Verification items for the finished model (mm, model axes). Round coordinates to 2 decimals unless told otherwise and drop trailing zeros. Loops run counter-clockwise (first coordinate to the right, second up) from the corner with the lowest first, then second, coordinate; pieces in that order, holes last. Notation, with made-up numbers: (76.25, -39) - (111.25, -39) arc R25 ccw to (111.25, -17) - close; hole circle Ø8 at (0.5, 43.25). An arc over 180 degrees is marked (long way). Use CSV: the item, a comma, the result in double quotes.
```python
from build123d import *

# Parameters (mm, degrees)
BOSS_EXTRUDE1_DEPTH = 76.2
SKETCH2_R           = 19.05
CUT_EXTRUDE1_DEPTH  = 140.97
SKETCH3_R           = 12.7
BOSS_EXTRUDE2_DEPTH = 50.8
SKETCH4_R           = 12.7
BOSS_EXTRUDE3_DEPTH = 50.8


with BuildPart() as part:
    # Sketch1 → Boss-Extrude1 (new body)
    with BuildSketch(Plane.XY):
        Polygon((0, 0), (533.4, 0), (533.4, 76.2), (25.4, 1471.918529083), (63.5, 1471.918529083), (63.5, 1535.418529083), (-63.5, 1535.418529083), (-63.5, 1471.918529083), (-25.4, 1471.918529083), (-533.4, 76.2), (-533.4, 0), align=None)
        Polygon((-452.309653737, 76.2), (452.309653737, 76.2), (0, 1318.910560245), align=None, mode=Mode.SUBTRACT)
    extrude(amount=BOSS_EXTRUDE1_DEPTH)

    # Sketch2 → Cut-Extrude1 (cut)
    with BuildSketch(Plane(origin=(63.5, 0, 0), x_dir=(0, 0, -1), z_dir=(1, 0, 0))):
        with Locations((-38.1, 1503.668529083)):
            Circle(SKETCH2_R)
    extrude(amount=-CUT_EXTRUDE1_DEPTH, mode=Mode.SUBTRACT)

    # Sketch3 → Boss-Extrude2 (add)
    with BuildSketch(Plane.ZY.offset(533.4)):
        with Locations((38.1, 38.1)):
            Circle(SKETCH3_R)
    extrude(amount=BOSS_EXTRUDE2_DEPTH)

    # Sketch4 → Boss-Extrude3 (add)
    with BuildSketch(Plane(origin=(533.4, 0, 0), x_dir=(0, 0, -1), z_dir=(1, 0, 0))):
        with Locations((-38.1, 38.1)):
            Circle(SKETCH4_R)
    extrude(amount=BOSS_EXTRUDE3_DEPTH)


solid = part.part
```
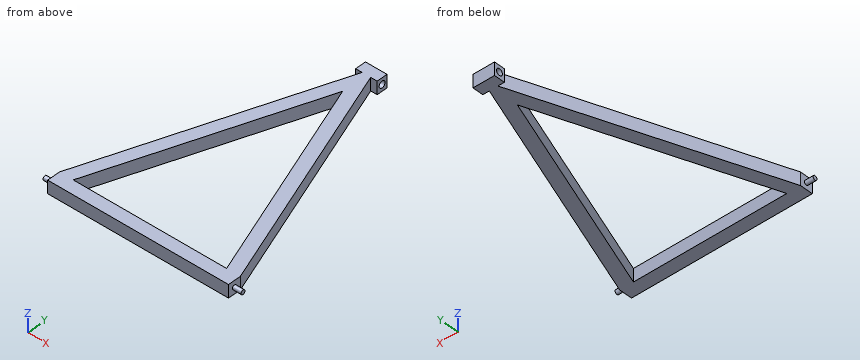
1) Cross-section at B-B, the plane y = 1102. Record the cut outline in (x, z), then the cut area to 3 significant figures.
Returned:
outline,"(-160.04, 0) - (-78.95, 0) - (-78.95, 76.2) - (-160.04, 76.2) - close; (78.95, 0) - (160.04, 0) - (160.04, 76.2) - (78.95, 76.2) - close"
area,"12,400 mm²"
2) Cross-section at C-C, the plane x = -266.5. Record the cut outline in (y, z).
Returned:
outline,"(0, 0) - (76.2, 0) - (76.2, 76.2) - (0, 76.2) - close; (586.71, 0) - (809.5, 0) - (809.5, 76.2) - (586.71, 76.2) - close"
3) Gauge pin test, flat ends, axial feed: pin 1 Ø6 at (y, z) = (1372, 48) entering from +X; pin 2 Ø5 at (y, z) = (629.5, 48) entering from -X; pin 3 Ø1.5 at (y, z) = (181.5, 28) entering from +X. Record the tip position at first contact, or that the pin passes through.
Returned:
pin 1,"stops at x = 62.86"
pin 2,"stops at x = -332.93"
pin 3,"stops at x = 495.35"
4) Cross-section at A-A, the plane z = 38.1. Record the cut outline in (x, y), then the cut area to 3 significant figures.
Returned:
outline,"(-584.2, 25.4) - (-533.4, 25.4) - (-533.4, 0) - (533.4, 0) - (533.4, 25.4) - (584.2, 25.4) - (584.2, 50.8) - (533.4, 50.8) - (533.4, 76.2) - (25.4, 1471.92) - (63.5, 1471.92) - (63.5, 1484.62) - (-63.5, 1484.62) - (-63.5, 1471.92) - (-25.4, 1471.92) - (-533.4, 76.2) - (-533.4, 50.8) - (-584.2, 50.8) - close; (-63.5, 1522.72) - (63.5, 1522.72) - (63.5, 1535.42) - (-63.5, 1535.42) - close; hole (-452.31, 76.2) - (452.31, 76.2) - (0, 1318.91) - close"
area,"305,000 mm²"
5) Thickness scan on probe 1 along X at (y, z) = (451, 32); probe 2 along X at (y, z) = (938, 36); probe 3 along X at (y, z) = (1458.5, 72). Record the ranges inside material, lowest first. Write a range as [from, to].
Returned:
probe 1,"x = [-396.98, -315.89], [315.89, 396.98]"
probe 2,"x = [-219.73, -138.64], [138.64, 219.73]"
probe 3,"x = [-30.28, 30.28]"
